For this review, take the finished solid that the model builds, in its own axes (mm). Face numbers are marked on the shaded views. A direction names the side the tool comes from. Round coordinates to 2 decimals unless told otherwise and drop trailing zeros. Loops run counter-clockwise (first coordinate to the right, second up) from the corner with the lowest first, then second, coordinate; pieces in that order, holes last.
1. Consider section A-A on x = 41. State the section outline as (y, z) points.
2. To check wall thickness, follow line 1 along Z through (x, y) = (80, -15); line 2 along Y through (x, z) = (81, 6.5); line 3 along Z through (x, y) = (15.5, 11). State the ranges of each line that lie inside material, in increasing order.
3. Consider section B-B on x = 15.5. State the section outline as (y, z) points.
4. Tool access review of the marked faces 4, 5 and 6: name each direction out of +Z, -Z, +X, -X, +Y, -Y from which nothing blocks a thin tool from reaching the whole face with its end or side.
5. Consider section C-C on x = 54. State the section outline as (y, z) points.
6. Clearance check with flat-ended pins moving along their axes: pin 1 Ø2.5 at (y, z) = (16.5, 6) entering from +X; pin 2 Ø1 at (x, y) = (59, 2) entering from +Z; pin 3 Ø0.6 at (x, y) = (68, 20.5) entering from -Z. State where each tip first meets the part, or that it passes through.
7. Consider section D-D on z = -37.5. State the section outline as (x, y) points, then the cut area to 3 significant figures.
8. Draft analysis for pull direction Y (two halves, no side actions). For the marked faces 1, 2 and 3, state which applies: released by +Y, released by -Y, zero draft, split by the parting line, or undercut.
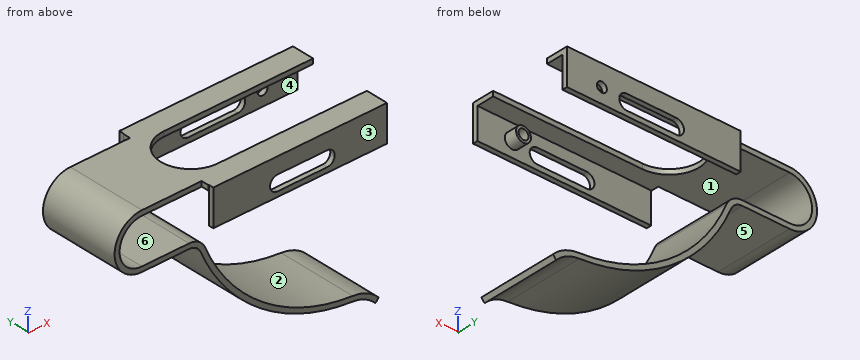
from build123d import *

# Parameters (mm, degrees)
F1_DEPTH  = 16
F3_W      = 70
F3_H      = 3
F4_DEPTH  = 2
F5_W      = 69.8145667315
F5_H      = 14.4820966907
F6_DEPTH  = 2
F9_DEPTH  = 2
F11_DEPTH = 42.001
F13_D     = 4
F13_DEPTH = 21.001
F14_R     = 3
F14_R_2   = 2
F15_DEPTH = 5


with BuildPart() as f1:
    # F0 (on Front) → F1 (new body)
    with BuildSketch(Plane.XZ):
        with BuildLine():
            Line((94, 11), (0, 11))
            ThreePointArc((0, 11), (-11, 0), (0, -11))
            Line((0, -11), (19, -11))
            ThreePointArc((19, -11), (21.7681124643, -11.8361612201), (23.6103896104, -14.064978646))
            ThreePointArc((23.6103896104, -14.064978646), (47.8977113224, -44.6078392712), (84.5520957277, -57.9942665386))
            ThreePointArc((84.5520957277, -57.9942665386), (89.6419160729, -59.3768457194), (93.8590048523, -62.5444881493))
            Line((93.8590048523, -62.5444881493), (95.1549842887, -61))
            ThreePointArc((95.1549842887, -61), (90.3976747979, -57.5207528796), (84.7034264019, -56))
            ThreePointArc((84.7034264019, -56), (49.0672193413, -42.9854179344), (25.4545454545, -13.2909701044))
            ThreePointArc((25.4545454545, -13.2909701044), (22.87535745, -10.1706257081), (19, -9))
            Line((19, -9), (0, -9))
            ThreePointArc((0, -9), (-9, 0), (0, 9))
            Line((0, 9), (94, 9))
            Line((94, 9), (94, 11))
        make_face()
    extrude(amount=F1_DEPTH)

    # F3 (on face) → F4 (join)
    with BuildSketch(Plane.XY.offset(11)):
        with Locations((59, -17.5)):
            Rectangle(F3_W, F3_H)
    extrude(amount=-F4_DEPTH)

    # F5 (on face) → F6 (join)
    with BuildSketch(Plane.XZ.offset(19)):
        with Locations((59.0927166343, 3.7589516547)):
            Rectangle(F5_W, F5_H)
    extrude(amount=F6_DEPTH)

    # F7: F1 across face


with BuildPart() as f1_1:
    add(f1.part)
    add(f1.part.mirror(Plane.XZ))

    # F8 (on face) → F9 (cut)
    with BuildSketch(Plane.XY.offset(11)):
        with BuildLine():
            Line((94, 12), (34, 12))
            ThreePointArc((34, 12), (22, 0), (34, -12))
            Line((34, -12), (94, -12))
            Line((94, -12), (94, 12))
        make_face()
    extrude(amount=-F9_DEPTH, mode=Mode.SUBTRACT)

    # F10 (on face) → F11 (cut, through all)
    with BuildSketch(Plane.XZ.offset(21)):
        with BuildLine():
            ThreePointArc((50, 4.5179033093), (47, 1.5179033093), (50, -1.4820966907))
            Line((50, -1.4820966907), (70, -1.4820966907))
            ThreePointArc((70, -1.4820966907), (73, 1.5179033093), (70, 4.5179033093))
            Line((70, 4.5179033093), (50, 4.5179033093))
        make_face()
    extrude(amount=-F11_DEPTH, mode=Mode.SUBTRACT)

    # F13 (through all, one way)
    with BuildSketch(Plane.XZ):
        with Locations((80, 2.5179033093)):
            Circle(F13_D / 2)
    extrude(amount=-F13_DEPTH, mode=Mode.SUBTRACT)

    # F14 (on face) → F15 (join)
    with BuildSketch(Plane(origin=(0, -19, 0), x_dir=(-1, 0, 0), z_dir=(0, 1, 0))):
        with Locations((-80, 2.5179033093)):
            Circle(F14_R)
        with Locations((-80, 2.5179033093)):
            Circle(F14_R_2, mode=Mode.SUBTRACT)
    extrude(amount=F15_DEPTH)


solid = f1_1.part
Resolved:
1. outline: (-21, -3.48) - (-19, -3.48) - (-19, 9) - (-12, 9) - (-12, 11) - (-21, 11) - close; (-16, -38.95) - (16, -38.95) - (16, -36.19) - (-16, -36.19) - close; (12, 9) - (19, 9) - (19, -3.48) - (21, -3.48) - (21, 11) - (12, 11) - close
2. line 1: z = -57.5 to -55.48, -0.48 to 0.52, 4.52 to 5.52, 9 to 11
2. line 2: y = -21 to -19, 19 to 21
2. line 3: z = -11 to -9, 9 to 11
3. outline: (-16, -11) - (16, -11) - (16, -9) - (-16, -9) - close; (-16, 9) - (16, 9) - (16, 11) - (-16, 11) - close
4. face 4: -Z, +X, -X
4. face 5: -Z, -X, +Y, -Y
4. face 6: +X, +Y, -Y
5. outline: (-21, -3.48) - (-19, -3.48) - (-19, -1.48) - (-21, -1.48) - close; (-21, 4.52) - (-19, 4.52) - (-19, 9) - (-12, 9) - (-12, 11) - (-21, 11) - close; (-16, -48.55) - (16, -48.55) - (16, -46.23) - (-16, -46.23) - close; (12, 9) - (19, 9) - (19, 4.52) - (21, 4.52) - (21, 11) - (12, 11) - close; (19, -3.48) - (21, -3.48) - (21, -1.48) - (19, -1.48) - close
6. pin 1: stops at x = -5.47
6. pin 2: stops at z = -48.71
6. pin 3: stops at z = -3.48
7. outline: (39.48, -16) - (42.37, -16) - (42.37, 16) - (39.48, 16) - close
7. area: 92.6 mm2
8. face 1: undercut
8. face 2: zero draft
8. face 3: released by -Y
